Could you check a few things on this drawing? It's one solid part, dimensions in mm from its lowest x, y, z. Give positions to 0.01 mm unless a question says otherwise; leave off trailing zeros. Order: outer loops, then holes, each group sorted by start corner. A loop starts at its lowest first (then second) coordinate and runs counter-clockwise, first axis right, second up. Notation, with made-up numbers: (-26.75, 10) -> (24.25, 10) arc R20 cw to (24.25, 31) -> close; hole circle Ø2 at (-31.75, 33). An arc over 180 degrees is marked (long way). Answer as a JSON object with one key per item and string values.
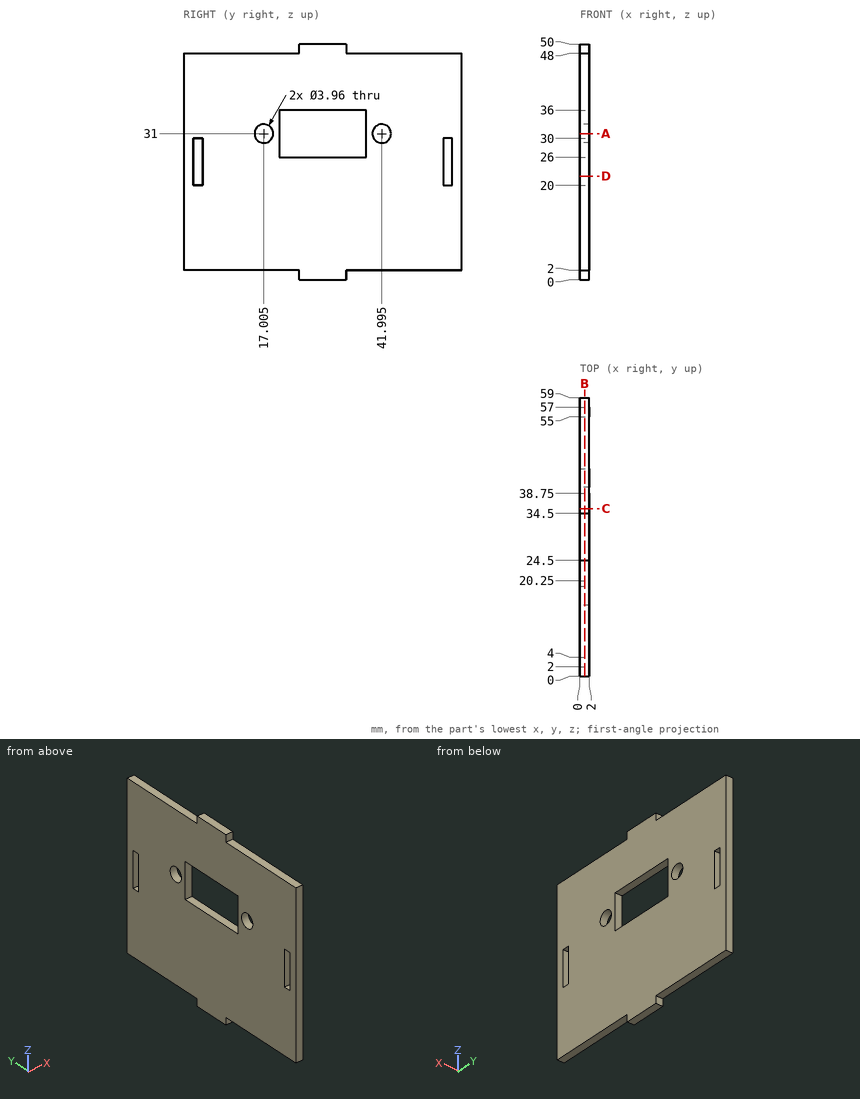
1. If we section it at C-C on y = 35.5: Please give me the cut outline in (x, z), then the cut area to 3 significant figures.
Worked answers:
{"outline": "(0, 2) -> (2, 2) -> (2, 26) -> (0, 26) -> close; (0, 36) -> (2, 36) -> (2, 48) -> (0, 48) -> close", "area": "72.0 mm²"}
2. If we section it at A-A on z = 31: Please give me the cut outline in (x, y) (3 decimals).
Worked answers:
{"outline": "(0, 0) -> (2, 0) -> (2, 15.025) -> (0, 15.025) -> close; (0, 18.985) -> (2, 18.985) -> (2, 20.25) -> (0, 20.25) -> close; (0, 38.75) -> (2, 38.75) -> (2, 40.015) -> (0, 40.015) -> close; (0, 43.975) -> (2, 43.975) -> (2, 59) -> (0, 59) -> close"}
3. If we section it at B-B on x = 1: Please give me the cut outline in (y, z) (3 decimals), then the cut area to 3 significant figures.
Worked answers:
{"outline": "(0, 2) -> (24.5, 2) -> (24.5, 0) -> (34.5, 0) -> (34.5, 2) -> (59, 2) -> (59, 48) -> (34.5, 48) -> (34.5, 50) -> (24.5, 50) -> (24.5, 48) -> (0, 48) -> close; hole (2, 20) -> (4, 20) -> (4, 30) -> (2, 30) -> close; hole circle Ø3.96 at (17.005, 31); hole (20.25, 26) -> (38.75, 26) -> (38.75, 36) -> (20.25, 36) -> close; hole circle Ø3.96 at (41.995, 31); hole (55, 20) -> (57, 20) -> (57, 30) -> (55, 30) -> close", "area": "2,500 mm²"}
4. Will these pins go through, and if not, where does the flat tip stop? pin 1 Ø1 at (x, y) = (1, 50) entering from -Z; pin 2 Ø0.6 at (x, z) = (1, 49.5) entering from -Y; pin 3 Ø1 at (x, y) = (1, 45) entering from +Z.
Worked answers:
{"pin 1": "z = 2", "pin 2": "y = 24.5", "pin 3": "z = 48"}
5. If we section it at D-D on z = 22: Please give me the cut outline in (x, y), then the cut area to 3 significant figures.
Worked answers:
{"outline": "(0, 0) -> (2, 0) -> (2, 2) -> (0, 2) -> close; (0, 4) -> (2, 4) -> (2, 55) -> (0, 55) -> close; (0, 57) -> (2, 57) -> (2, 59) -> (0, 59) -> close", "area": "110 mm²"}
6. Please list where these lines run through material, in increasing order: L1, parallel to Y at x = 1.4, z = 22.5; L2, parallel to Z at x = 0.35, y = 3.5; L3, parallel to Z at x = 1.6, y = 42.
Worked answers:
{"L1": "0 to 2, 4 to 55, 57 to 59", "L2": "2 to 20, 30 to 48", "L3": "2 to 29.02, 32.98 to 48"}
